Source: CAD feature listing. Evaluate the final solid. Frame: model axes, mm. A direction names the side the tool comes from. Coordinates: 2 decimals unless noted, no trailing zeros. Loops run counter-clockwise (first coordinate to the right, second up) from the corner with the lowest first, then second, coordinate; pieces in that order, holes last.
from build123d import *

# Parameters (mm, degrees)
CROQUIS1_R              = 62
SALIENTE_EXTRUIR1_DEPTH = 45
CROQUIS3_R              = 23.5
CORTAR_EXTRUIR1_DEPTH   = 8
CROQUIS4_R              = 20
CORTAR_EXTRUIR2_DEPTH   = 99.554553421
CORTAR_EXTRUIR3_DEPTH   = 99.554553421


with BuildPart() as part:
    # Croquis1 → Saliente-Extruir1 (new body)
    with BuildSketch(Plane(origin=(0, 0, 0), x_dir=(1, 0, 0), z_dir=(0, 1, 0))):
        with Locations(Location((0, 0, 0), (0, 0, 90))):
            Circle(CROQUIS1_R)
    extrude(amount=SALIENTE_EXTRUIR1_DEPTH)

    # Croquis3 → Cortar-Extruir1 (cut)
    with BuildSketch(Plane.XZ):
        with Locations(Location((0, 0, 0), (0, 0, 270))):
            Circle(CROQUIS3_R)
    extrude(amount=-CORTAR_EXTRUIR1_DEPTH, mode=Mode.SUBTRACT)

    # Croquis4 → Cortar-Extruir2 (cut, through all)
    with BuildSketch(Plane.XZ):
        with Locations(Location((0, 0, 0), (0, 0, 270))):
            Circle(CROQUIS4_R)
    extrude(amount=-CORTAR_EXTRUIR2_DEPTH, mode=Mode.SUBTRACT)

    # Croquis5 → Cortar-Extruir3 (cut, through all)
    with BuildSketch(Plane.XZ):
        with BuildLine():
            Line((0, 30), (0, 50))
            Line((0, 50), (36.66060556, 50))
            Line((36.66060556, 50), (110, 15))
            Line((110, 15), (110, -15))
            Line((110, -15), (36.66060556, -50))
            Line((36.66060556, -50), (0, -50))
            Line((0, -50), (0, -30))
            ThreePointArc((0, -30), (30, 0), (0, 30))
        make_face()
    extrude(amount=-CORTAR_EXTRUIR3_DEPTH, mode=Mode.SUBTRACT)


solid = part.part
Q1. Access query for faces 4 (the flat face through (-24, 45, 1)), 5 (the flat face through (19, 8, -7)), 6 (the flat face through (19, 22, -50)). Directions: +Z, -Z, +X, -X, +Y, -Y. A direction counts if a zero-diameter tool reaches every point of the face in a straight line with its end or side. Return the directions, or none.
Q2. Draft query along Z for faces 1 (the cylindrical face through (-19.524, 26.241, 4.336)), 2 (the cylindrical face through (-61.97, 22.18, -1.91)), 3 (the flat face through (-24, 0, 1)). Return one class per face: +Z half, -Z half, draft (parallel to the pull), parting line (faces both ways), or undercut.
Q3. Section B-B, the plane x = 22. Return the cut outline in (y, z), plus the area to 3 significant figures.
Q4. Section D-D, the plane z = -25. Return the cut outline in (x, y), plus the area to 3 significant figures.
Q5. Section A-A, the plane y = 34. Return the cut outline in (x, z), plus the area to 3 significant figures.
Q6. Section C-C, the plane z = 0. Return the cut outline in (x, y).
Q7. Line query: line 1 along X through (y, z) = (4, 0); line 2 along Z through (x, y) = (-7, 4); line 3 along X through (y, z) = (18, -3). Output: solid intervals per line, ascending.
Q8. Contact query for flat-ended pins moving along their axis: pin 1 Ø10 at (y, z) = (16.5, -41) entering from +X; pin 2 Ø3 at (x, z) = (-28.5, -24.5) entering from -Y; pin 3 Ø6 at (x, y) = (-4, 14.5) entering from +Z; pin 4 Ø24 at (x, z) = (0, 0) entering from -Y. Output: stop coordinate, or through.
Derived:
1. face 4: +Z, -Z, +X, -X, +Y
1. face 5: -Y
1. face 6: +X, +Y, -Y
2. face 1: undercut
2. face 2: parting line
2. face 3: draft
3. outline: (0, -57.97) - (45, -57.97) - (45, -50) - (0, -50) - close; (0, -20.4) - (45, -20.4) - (45, 20.4) - (0, 20.4) - (0, 8.26) - (8, 8.26) - (8, -8.26) - (0, -8.26) - close; (0, 50) - (45, 50) - (45, 57.97) - (0, 57.97) - close
3. area: 2,420 mm2
4. outline: (-56.74, 0) - (16.58, 0) - (16.58, 45) - (-56.74, 45) - close
4. area: 3,300 mm2
5. outline: (0, -50) - (0, -30) arc R30 ccw to (0, 30) - (0, 50) - (36.66, 50) arc R62 ccw (long way) to (36.66, -50) - close; hole circle Ø40 at (0, 0)
5. area: 6,790 mm2
6. outline: (-62, 0) - (-23.5, 0) - (-23.5, 8) - (-20, 8) - (-20, 45) - (-62, 45) - close; (20, 8) - (23.5, 8) - (23.5, 0) - (30, 0) - (30, 45) - (20, 45) - close
7. line 1: x = -62 to -23.5, 23.5 to 30
7. line 2: z = -61.6 to -22.43, 22.43 to 61.6
7. line 3: x = -61.93 to -19.77, 19.77 to 29.85
8. pin 1: stops at x = 0
8. pin 2: stops at y = 0
8. pin 3: stops at z = 61.99
8. pin 4: passes through
